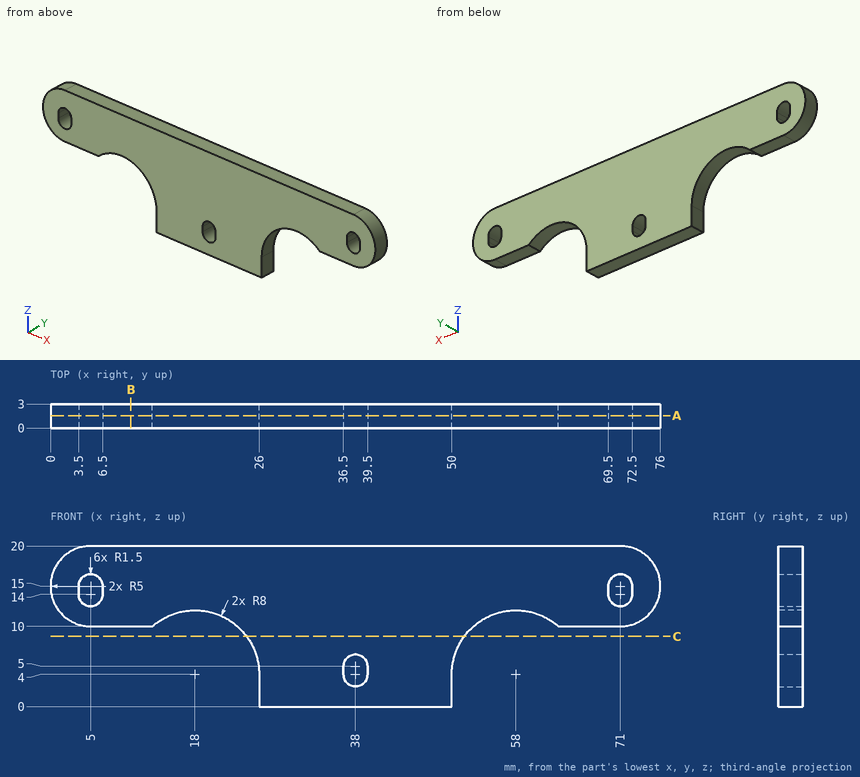
Part print with two shaded views. Sizes in mm from the minimum x, y, z corner. Round coordinates to 2 decimals unless told otherwise and drop trailing zeros. Order: outer loops, then holes, each group sorted by start corner. A loop starts at its lowest first (then second) coordinate and runs counter-clockwise, first axis right, second up. Notation, with made-up numbers: (89.5, 45.5) - (107.5, 45.5) arc R32 cw to (107.5, 71.5) - close; hole circle Ø7 at (33, 69). An arc over 180 degrees is marked (long way). Return JSON: item names as keys, results as strings.
(1) Cut at B-B (x = 10). Give the cut face in (y, z), then the cut area to 3 significant figures.
Answer key:
{"outline": "(0, 10) - (3, 10) - (3, 20) - (0, 20) - close", "area": "30.0 mm^2"}
(2) Pin check, flat tips, straight feed: pin 1 Ø0.8 at (y, z) = (2, 4.5) entering from -X; pin 2 Ø1.5 at (x, y) = (23.5, 0.5) entering from -Z; pin 3 Ø0.5 at (y, z) = (1.5, 14.5) entering from -X. Stop position of each tip, or through.
Answer key:
{"pin 1": "stops at x = 25.95", "pin 2": "stops at z = 8.99", "pin 3": "stops at x = 0.01"}
(3) Cut at A-A (y = 1.55). Give the cut face in (x, z).
Answer key:
{"outline": "(5, 10) - (12.71, 10) arc R8 cw to (26, 4) - (26, 0) - (50, 0) - (50, 4) arc R8 cw to (63.29, 10) - (71, 10) arc R5 ccw to (71, 20) - (5, 20) arc R5 ccw to start; hole (3.5, 14) arc R1.5 ccw to (6.5, 14) - (6.5, 15) arc R1.5 ccw to (3.5, 15) - close; hole (36.5, 4) arc R1.5 ccw to (39.5, 4) - (39.5, 5) arc R1.5 ccw to (36.5, 5) - close; hole (69.5, 14) arc R1.5 ccw to (72.5, 14) - (72.5, 15) arc R1.5 ccw to (69.5, 15) - close"}
(4) Cut at C-C (z = 8.75). Give the cut face in (x, y).
Answer key:
{"outline": "(24.44, 0) - (51.56, 0) - (51.56, 3) - (24.44, 3) - close"}
(5) Wall check: probe 1 along X at (y, z) = (2.2, 10.75); probe 2 along Z at (x, y) = (38, 0.9); probe 3 along Z at (x, y) = (72, 1.95). Give the ranges that are in metal, low to high. Write a range as from..to.
Answer key:
{"probe 1": "x = 2.37..13.71, 22.29..53.71, 62.29..73.63", "probe 2": "z = 0..2.5, 6.5..20", "probe 3": "z = 10.1..12.88, 16.12..19.9"}
